from build123d import *

# Parameters (mm, degrees)
BOSS_EXTRUDE1_DEPTH = 6.35
SKETCH2_R           = 3.5
CUT_EXTRUDE1_DEPTH  = 7.35


with BuildPart() as part:
    # Sketch1 → Boss-Extrude1 (new body)
    with BuildSketch(Plane.XY):
        Polygon((12.7, 0), (-12.7, 0), (-12.7, 50.8), (-63.1, 50.8), (-63.1, 76.2), (12.7, 76.2), (12.7, 50.8), align=None)
    extrude(amount=BOSS_EXTRUDE1_DEPTH)

    # Sketch2 → Cut-Extrude1 (cut, through all)
    with BuildSketch(Plane.XY.offset(6.35)):
        with Locations((0, 63.5)):
            Circle(SKETCH2_R)
        with Locations((-25.4, 63.5)):
            Circle(SKETCH2_R)
        with Locations((0, 38.1)):
            Circle(SKETCH2_R)
        with Locations((0, 12.7)):
            Circle(SKETCH2_R)
        with Locations((-50.8, 63.5)):
            Circle(SKETCH2_R)
    extrude(amount=-CUT_EXTRUDE1_DEPTH, mode=Mode.SUBTRACT)


solid = part.part
The model under review builds one solid part; all positions refer to its coordinate system, in mm. A direction names the side the tool comes from. Round coordinates to 2 decimals unless told otherwise and drop trailing zeros. Loops run counter-clockwise (first coordinate to the right, second up) from the corner with the lowest first, then second, coordinate; pieces in that order, holes last. Notation, with made-up numbers: M 76,-22 L 93,-22 A23 cw 93,16 Z; hole C 25,81 d1. An arc over 180 degrees is marked long. Answer as a JSON object with one key per item and string values.
Item 1: We need section C-C, the plane x = 0. State the section outline as (y, z) points.
Check sheet entries:
{"outline": "M 0,0 L 9.2,0 L 9.2,6.35 L 0,6.35 Z; M 16.2,0 L 34.6,0 L 34.6,6.35 L 16.2,6.35 Z; M 41.6,0 L 60,0 L 60,6.35 L 41.6,6.35 Z; M 67,0 L 76.2,0 L 76.2,6.35 L 67,6.35 Z"}
Item 2: We need section D-D, the plane z = 2.5. State the section outline as (x, y) points, and give its area (3 significant figures).
Check sheet entries:
{"outline": "M -63.1,50.8 L -12.7,50.8 L -12.7,0 L 12.7,0 L 12.7,76.2 L -63.1,76.2 Z; hole C -50.8,63.5 d7; hole C -25.4,63.5 d7; hole C 0,12.7 d7; hole C 0,38.1 d7; hole C 0,63.5 d7", "area": "3,020 mm2"}
Item 3: Clearance check with flat-ended pins moving along their axes: P1, Ø1, axis at y = 20.5, z = 3, coming from the -X side; P2, Ø3, axis at x = -41, z = 4.5, coming from the -Y side. State where each tip first meets the part, or that it passes through.
Check sheet entries:
{"P1": "x = -12.7", "P2": "y = 50.8"}
Item 4: We need section B-B, the plane y = 12.7. State the section outline as (x, z) points, and give its area (3 significant figures).
Check sheet entries:
{"outline": "M -12.7,0 L -3.5,0 L -3.5,6.35 L -12.7,6.35 Z; M 3.5,0 L 12.7,0 L 12.7,6.35 L 3.5,6.35 Z", "area": "117 mm2"}
Item 5: We need section A-A, the plane x = -50.8. State the section outline as (y, z) points, and give its area (3 significant figures).
Check sheet entries:
{"outline": "M 50.8,0 L 60,0 L 60,6.35 L 50.8,6.35 Z; M 67,0 L 76.2,0 L 76.2,6.35 L 67,6.35 Z", "area": "117 mm2"}
Item 6: The part is to be moulded in two halves that separate along Y. For faces 1 (the face through (0, 0, 3)), 2 (the face through (-47.46, 64.55, 3.22)), 3 (the face through (-8, 47, 0)), say which applies: +Y half, -Y half, draft (parallel to the pull), parting line (faces both ways), or undercut.
Check sheet entries:
{"face 1": "-Y half", "face 2": "undercut", "face 3": "draft"}
Item 7: Tool access review of faces 4 (the face through (-26, 76.2, 3)), 5 (the face through (-38, 50.8, 3)): name each direction out of +Z, -Z, +X, -X, +Y, -Y from which nothing blocks a thin tool from reaching the whole face with its end or side.
Check sheet entries:
{"face 4": "+Z, -Z, +X, -X, +Y", "face 5": "+Z, -Z, -X, -Y"}
Item 8: For line 1 along Y through (x, z) = (0, 4); line 2 along Y through (x, z) = (3, 1); line 3 along X through (y, z) = (47, 0.5), list the stretches that pass through material, from the lowest coordinate up.
Check sheet entries:
{"line 1": "0 to 9.2, 16.2 to 34.6, 41.6 to 60, 67 to 76.2", "line 2": "0 to 10.9, 14.5 to 36.3, 39.9 to 61.7, 65.3 to 76.2", "line 3": "-12.7 to 12.7"}
